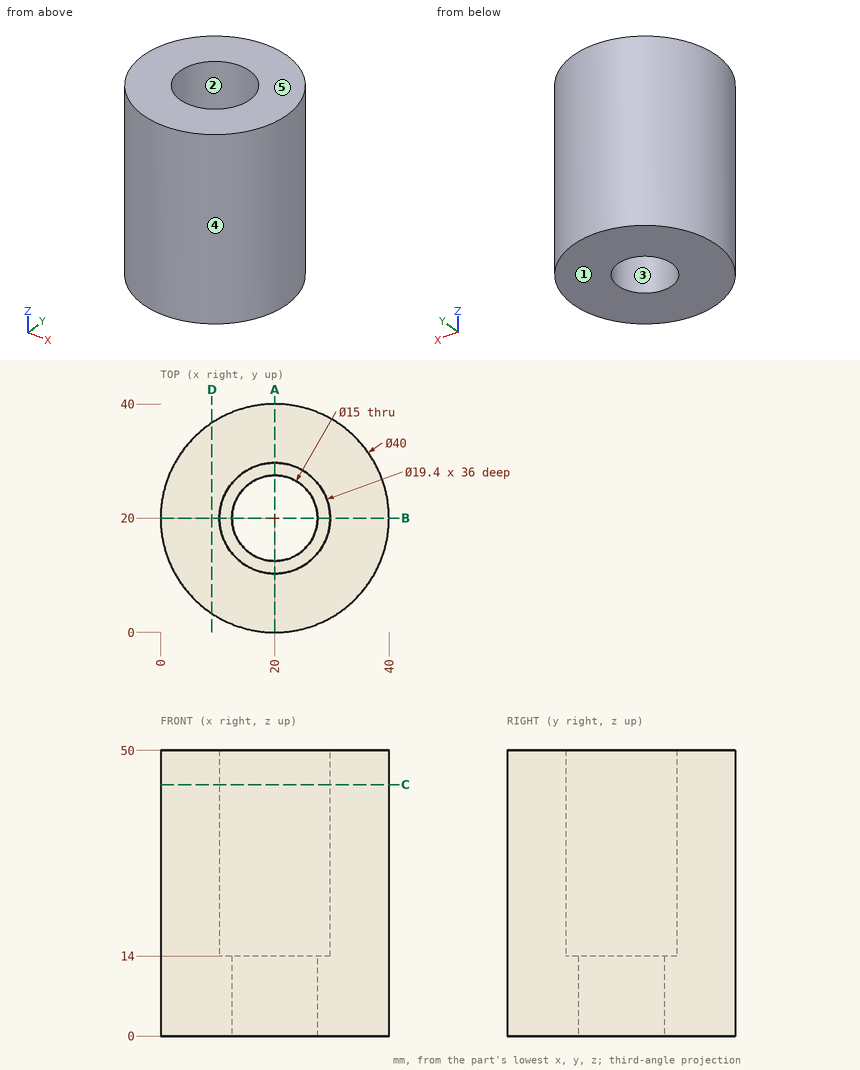
Answer from the drawing. Dimensions are ordinates in mm from the lowest x, y and z of the part. A direction names the side the tool comes from. Coordinates: 2 decimals unless noted, no trailing zeros. Loops run counter-clockwise (first coordinate to the right, second up) from the corner with the lowest first, then second, coordinate; pieces in that order, holes last. Notation, with made-up numbers: (84, 82) -> (140, 82) arc R10 ccw to (140, 87) -> close; hole circle Ø11 at (79.25, 81). An arc over 180 degrees is marked (long way). Answer in a Markdown table with one row per item.
Item 1: Straight lines are drawn through the part: line 1 along Y through (x, z) = (20, 4.25); line 2 along Y through (x, z) = (20, 37); line 3 along X through (y, z) = (18, 16.5). For each, find the intervals that lie inside material, in ascending order. Write a range as [from, to].
Returned:
| item | result |
|---|---|
| line 1 | y = [0, 12.5], [27.5, 40] |
| line 2 | y = [0, 10.3], [29.7, 40] |
| line 3 | x = [0.1, 10.51], [29.49, 39.9] |
Item 2: A cutting plane is placed at A-A on x = 20. Determine the outline of the cut face in (y, z), plus the area to 3 significant figures.
Returned:
| item | result |
|---|---|
| outline | (0, 0) -> (12.5, 0) -> (12.5, 14) -> (10.3, 14) -> (10.3, 50) -> (0, 50) -> close; (27.5, 0) -> (40, 0) -> (40, 50) -> (29.7, 50) -> (29.7, 14) -> (27.5, 14) -> close |
| area | 1,090 mm^2 |
Item 3: For the marked faces 1 and 2, determine the directions among +Z, -Z, +X, -X, +Y, -Y from which every point of the face is accessible in a straight line to the end or side of a thin tool.
Returned:
| item | result |
|---|---|
| face 1 | -Z, +X, -X, +Y, -Y |
| face 2 | +Z |
Item 4: Each of these flat-tipped pins is pushed along its axis until it touches: P1, Ø8, axis at x = 8.5, z = 10.5, coming from the +Y side; P2, Ø1.5, axis at y = 5.5, z = 35.5, coming from the -X side; P3, Ø2, axis at x = 22, z = 37, coming from the +Y side (3 decimals). Where does it stop, or does it pass through?
Returned:
| item | result |
|---|---|
| P1 | stops at y = 38.54 |
| P2 | stops at x = 5.48 |
| P3 | stops at y = 39.975 |
Item 5: For a pull along Y with two mould halves and no side action, classify the marked faces 3, 4 and 5 as released by +Y, released by -Y, zero draft, split by the parting line, or undercut.
Returned:
| item | result |
|---|---|
| face 3 | undercut |
| face 4 | split by the parting line |
| face 5 | zero draft |
Item 6: A cutting plane is placed at D-D on x = 9. Determine the outline of the cut face in (y, z), plus the area to 3 significant figures.
Returned:
| item | result |
|---|---|
| outline | (3.3, 0) -> (36.7, 0) -> (36.7, 50) -> (3.3, 50) -> close |
| area | 1,670 mm^2 |
Item 7: A cutting plane is placed at C-C on z = 44. Determine the outline of the cut face in (x, y), plus the area to 3 significant figures.
Returned:
| item | result |
|---|---|
| outline | circle Ø40 at (20, 20); hole circle Ø19.4 at (20, 20) |
| area | 961 mm^2 |
